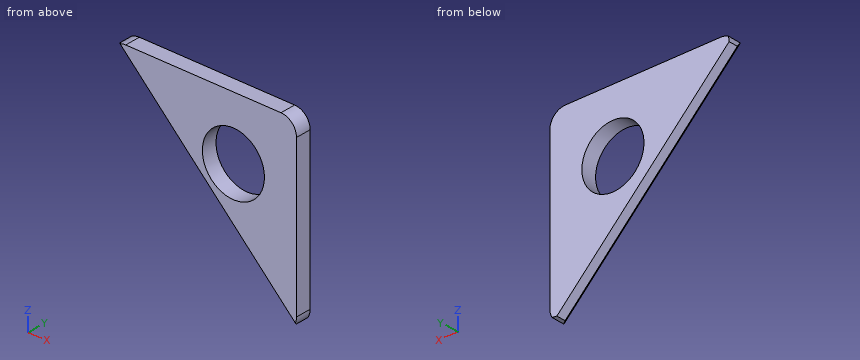
from build123d import *

# Parameters (mm, degrees)
F0_R        = 50
F1_DEPTH    = 25
F2_SIZE     = 10
F3_T1_DEPTH = 47.2159409701


# Not quite as in the source:
# - a fillet or chamfer that OpenCascade refuses, or shapes differently, is made with other operations: its cross-section is extruded or revolved along the edge and cut away or added


with BuildPart() as f1:
    # F0 (on Front) → F1 (new body)
    with BuildSketch(Plane.XZ):
        with BuildLine():
            Line((51.0779787002, 143.0251310061), (-198.9220212998, 143.0251310061))
            ThreePointArc((-198.9220212998, 143.0251310061), (-208.4891071089, 141.1221193189), (-216.5996908295, 135.7028005358))
            Line((-216.5996908295, 135.7028005358), (68.7556482299, -149.6525385235))
            ThreePointArc((68.7556482299, -149.6525385235), (74.174967013, -141.541954803), (76.0779787002, -131.9748689939))
            Line((76.0779787002, -131.9748689939), (76.0779787002, 118.0251310061))
            ThreePointArc((76.0779787002, 118.0251310061), (68.7556482299, 135.7028005358), (51.0779787002, 143.0251310061))
        make_face()
        with Locations((-25.4944633545, 42.9471413087)):
            Circle(F0_R, mode=Mode.SUBTRACT)
    extrude(amount=F1_DEPTH)

    # F2
    f2_edges = [f1.edges().sort_by_distance(p)[0] for p in [
        (-73.922021, -25, -6.974869),
    ]]
    chamfer(f2_edges, length=F2_SIZE)

    # F3: chamfer of 5 on 2 edges, made by hand

    # F3_s2 → F3_t1 (cut)
    with BuildSketch(Plane.XZ.offset(-16.1079704851)):
        with BuildLine():
            Line((64.7710426378, -145.6679329315), (72.6137260047, -144.6717815335))
            ThreePointArc((72.6137260047, -144.6717815335), (70.8856590953, -147.2279276171), (68.7556482299, -149.6525385235))
            Line((68.7556482299, -149.6525385235), (64.7710426378, -145.6679329315))
        make_face()
        with BuildLine():
            Line((-211.6189338394, 139.5608783106), (-212.6150852374, 131.7181949438))
            Line((-212.6150852374, 131.7181949438), (-216.5996908295, 135.7028005358))
            ThreePointArc((-216.5996908295, 135.7028005358), (-214.1750799231, 137.8328114012), (-211.6189338394, 139.5608783106))
        make_face()
    extrude(amount=F3_T1_DEPTH, mode=Mode.SUBTRACT)


solid = f1.part
Input: part model. Units: mm. Frame: model coordinates. Give positions to 0.01 mm unless a question says otherwise; leave off trailing zeros. Order: outer loops, then holes, each group sorted by start corner. A loop starts at its lowest first (then second) coordinate and runs counter-clockwise, first axis right, second up. Notation, with made-up numbers: (34.5, 50.25) - (89.5, 50.25) arc R15 cw to (89.5, 63.25) - close; hole circle Ø6 at (35, 56.25). An arc over 180 degrees is marked (long way). Write each question's results on one line, items separated by ' | '.
Item 1: Section C-C (y = -7). Return loops of the section in (x, z).
A:
outline: (-212.62, 131.72) - (64.77, -145.67) - (72.61, -144.67) arc R25 ccw to (76.08, -131.97) - (76.08, 118.03) arc R25 ccw to (51.08, 143.03) - (-198.92, 143.03) arc R25 ccw to (-211.62, 139.56) - close; hole circle Ø100 at (-25.49, 42.95)
Item 2: Contact query for flat-ended pins moving along their axis: pin 1 Ø4 at (y, z) = (-11, 17.5) entering from -X; pin 2 Ø10 at (y, z) = (-14.5, -64.5) entering from -X; pin 3 Ø1 at (x, y) = (-46.5, -18) entering from -Z. Output: stop coordinate, or through.
A:
pin 1: stops at x = -100.4 | pin 2: stops at x = -21.4 | pin 3: stops at z = -31.02
Item 3: Section A-A (z = 33). Return loops of the section in (x, y).
A:
outline: (-113.9, -15) - (-99.75, -25) - (-74.5, -25) - (-74.5, 0) - (-113.9, 0) - close; (23.51, -25) - (76.08, -25) - (76.08, 0) - (23.51, 0) - close
Item 4: Material intervals for line 1 along X through (y, z) = (-8.5, 77); line 2 along Z through (x, y) = (-69.5, -1.5); line 3 along X through (y, z) = (-17.5, 15), sorted ascending.
A:
line 1: x = -157.9 to -62.11, 11.12 to 76.08 | line 2: z = -11.4 to 19.21, 66.69 to 143.03 | line 3: x = -92.36 to -66.95, 15.97 to 76.08
Item 5: Section D-D (z = -96). Return loops of the section in (x, y), and give its area (3 significant figures).
A:
outline: (15.1, -15) - (29.25, -25) - (76.08, -25) - (76.08, 0) - (15.1, 0) - close | area: 1,450 mm^2
Item 6: Section B-B (x = -24.5). Return loops of the section in (y, z), and give its area (3 significant figures).
A:
outline: (-25, -42.25) - (-15, -56.4) - (0, -56.4) - (0, -7.04) - (-25, -7.04) - close; (-25, 92.94) - (0, 92.94) - (0, 143.03) - (-25, 143.03) - close | area: 2,420 mm^2
